The figure shows three views and two pictorial views of one solid part (mm, origin at its lowest corner). Answer the questions. A direction names the side the tool comes from. Give positions to 0.01 mm unless a question says otherwise; leave off trailing zeros. Loops run counter-clockwise (first coordinate to the right, second up) from the corner with the lowest first, then second, coordinate; pieces in that order, holes last. Notation, with made-up numbers: M 33.5,40 L 68.5,40 A34 cw 68.5,72 Z; hole C -34.75,66.25 d1. An arc over 180 degrees is marked long. Answer as a JSON object with one key per item and string values. Group by question number.
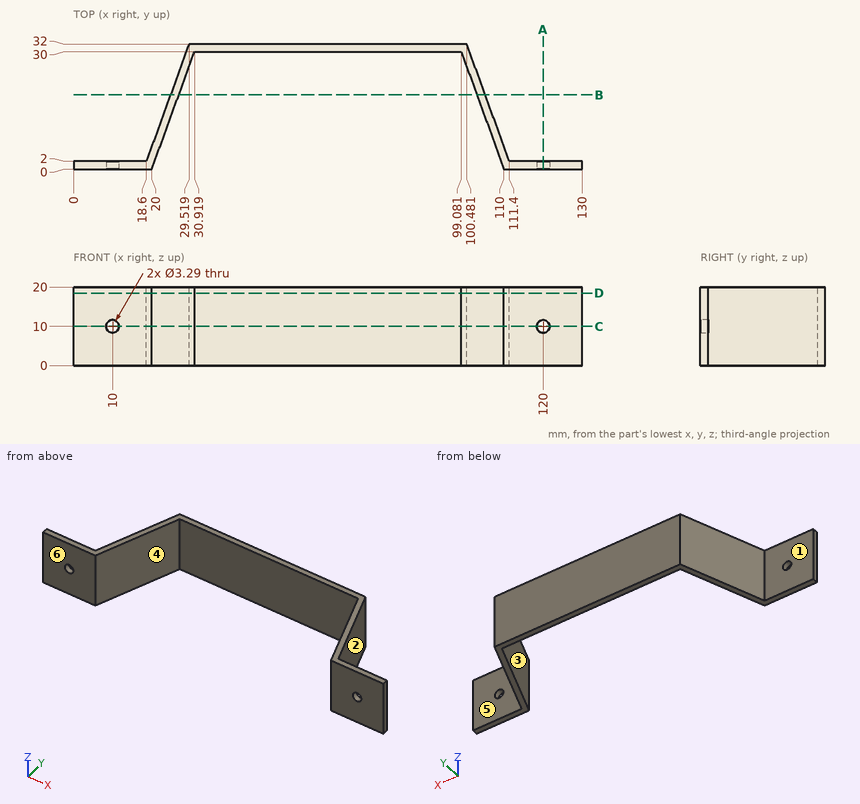
Item 1: For a pull along X with two mould halves and no side action, classify the marked faces 1, 2 and 3 as pulls with the +X half, pulls with the -X half, needs draft (parallel to the pull), parting line crosses it, or undercut.
Item 2: A cutting plane is placed at A-A (x = 120). Determine the outline of the cut face in (y, z) (1 decimal).
Item 3: Given pin 1 Ø4 at (y, z) = (16, 7) entering from -X; pin 2 Ø2 at (y, z) = (28, 12) entering from +X; pin 3 Ø9.5 at (x, z) = (117, 12.5) entering from +Y; pin 4 Ø4.5 at (x, z) = (10, 10) entering from -Y, each flat-ended and moving along its own axis, determine where each tip first touches the part or whether it passes through.
Item 4: A cutting plane is placed at B-B (y = 19). Determine the outline of the cut face in (x, z) (1 decimal).
Item 5: A tool of negligible diameter and unlimited length cuts with its end or side. For the marked faces 4, 5 and 6, from which of +Z, -Z, +X, -X, +Y, -Y can it reach the whole face along a straight path? Write none if from no direction.
Item 6: A cutting plane is placed at D-D (z = 18.5). Determine the outline of the cut face in (x, y), and give its area (3 significant figures).
Item 7: Find the intervals of material crossed by probe 1 along X at (y, z) = (1.05, 10) (1 decimal); probe 2 along X at (y, z) = (0.6, 10) (1 decimal); probe 3 along Z at (x, y) = (10, 1) (1 decimal), in increasing order. Write a range as [from, to].
Item 8: A cutting plane is placed at C-C (z = 10). Determine the outline of the cut face in (x, y) (1 decimal), and give its area (3 significant figures).
The answers:
{
 "1": {"face 1": "needs draft", "face 2": "pulls with the +X half", "face 3": "undercut"},
 "2": {"outline": "M 0,0 L 2,0 L 2,8.4 L 0,8.4 Z; M 0,11.6 L 2,11.6 L 2,20 L 0,20 Z"},
 "3": {"pin 1": "stops at x = 22.97", "pin 2": "stops at x = 102.3", "pin 3": "stops at y = 2", "pin 4": "stops at y = 0"},
 "4": {"outline": "M 24.8,0 L 26.9,0 L 26.9,20 L 24.8,20 Z; M 103.1,0 L 105.2,0 L 105.2,20 L 103.1,20 Z"},
 "5": {"face 4": "+Z, -Z, -Y", "face 5": "+Z, -Z, +X, +Y", "face 6": "+Z, -Z, +X, -X, -Y"},
 "6": {"outline": "M 0,0 L 20,0 L 30.92,30 L 99.08,30 L 110,0 L 130,0 L 130,2 L 111.4,2 L 100.48,32 L 29.52,32 L 18.6,2 L 0,2 Z", "area": "344 mm^2"},
 "7": {"probe 1": "x = [0, 8.4], [11.6, 20.4], [109.6, 118.4], [121.6, 130]", "probe 2": "x = [0, 8.4], [11.6, 20.2], [109.8, 118.4], [121.6, 130]", "probe 3": "z = [0, 8.4], [11.6, 20]"},
 "8": {"outline": "M 0,0 L 8.4,0 L 8.4,2 L 0,2 Z; M 11.6,0 L 20,0 L 30.9,30 L 99.1,30 L 110,0 L 118.4,0 L 118.4,2 L 111.4,2 L 100.5,32 L 29.5,32 L 18.6,2 L 11.6,2 Z; M 121.6,0 L 130,0 L 130,2 L 121.6,2 Z", "area": "331 mm^2"}
}
